Design review of the part built by this model. Coordinates are the model's own, in mm. Face numbers are marked on the shaded views. A direction names the side the tool comes from. Coordinates: 2 decimals unless noted, no trailing zeros. Loops run counter-clockwise (first coordinate to the right, second up) from the corner with the lowest first, then second, coordinate; pieces in that order, holes last. Notation, with made-up numbers: (-32.75, 68.5) -> (-19.75, 68.5) arc R23 ccw to (-19.75, 104.5) -> close; hole circle Ø6 at (82, -18). An arc over 180 degrees is marked (long way). One line per item, written item: value. Start each with the question number.
1. Insertion check: pin 1 (3 mm diameter, centred on x = -8, y = 11, fed in from -Z); pin 2 (4 mm diameter, centred on x = -7.5, y = 8.5, fed in from +Z). Each pin has a flat end and moves straight along its axis. Give the tip position at first contact, or say it passes through.
2. Draft analysis for pull direction Y (two halves, no side actions). For the marked faces 3, 4 and 5, state which applies: pulls with the +Y half, pulls with the -Y half, needs draft (parallel to the pull), parting line crosses it, or undercut.
3. For probe 1 along Y at (x, z) = (-3.75, -1.5); probe 2 along X at (y, z) = (14, -2.25); probe 3 along X at (y, z) = (18, 0.5), list the stretches that pass through material, from the lowest coordinate up.
4. Add section A-A on y = 31.5. Write out the cut boundary in (x, z).
5. Machinability: for the marked faces 1 and 2, which of the approach directions +Z, -Z, +X, -X, +Y, -Y give a long, thin tool a straight path to every point of the face, cutting with its end or side? Answer none if there is none.
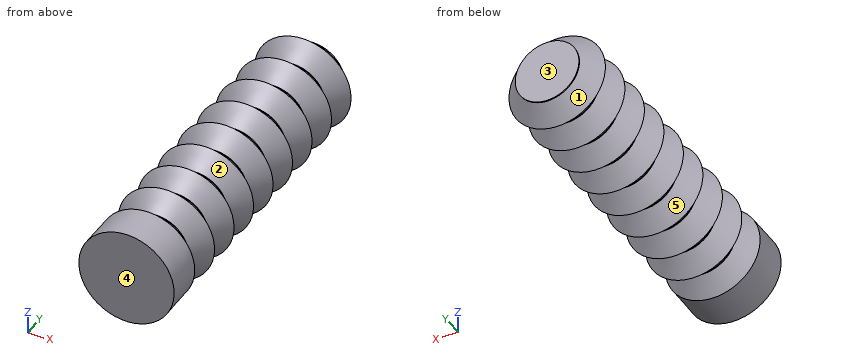
```python
from build123d import *


# Read off the part's stored shape, not the designer's step: Thicken1
with BuildPart() as part:
    # Thicken1 outline → Thicken1 (revolve)
    with BuildSketch(Plane(origin=(-5.431630681, 0, 0), x_dir=(1, 0, 0), z_dir=(0, 0, 1))):
        Polygon((0, -0.954433192), (0, -1.754433192), (4.941383818, -1.754433192), (4.918558927, 2.245501685), (3.3, 3.988409531), (3.3, 4.088409531), (5, 5.913409531), (3.3, 7.738409531), (3.3, 7.838409531), (5, 9.663409531), (3.3, 11.488409531), (3.3, 11.588409531), (5, 13.413409531), (3.3, 15.238409531), (3.3, 15.338409531), (5, 17.163409531), (3.3, 18.988409531), (3.3, 19.088409531), (5, 20.913409531), (3.3, 22.738409531), (3.3, 22.838409531), (5, 24.663409531), (3.3, 26.488409531), (3.3, 26.588409531), (5, 28.413409531), (3.3, 30.238409531), (3.3, 30.338409531), (5, 32.163409531), (3.3, 33.988409531), (3.3, 34.102954004), (0, 34.102954004), (0, 33.302954004), (2.845194483, 33.302954004), (3.906687965, 32.163409531), (2.5, 30.653288628), (2.5, 29.923530434), (3.906687965, 28.413409531), (2.5, 26.903288628), (2.5, 26.173530434), (3.906687965, 24.663409531), (2.5, 23.153288628), (2.5, 22.423530434), (3.906687965, 20.913409531), (2.5, 19.403288628), (2.5, 18.673530434), (3.906687965, 17.163409531), (2.5, 15.653288628), (2.5, 14.923530434), (3.906687965, 13.413409531), (2.5, 11.903288628), (2.5, 11.173530434), (3.906687965, 9.663409531), (2.5, 8.153288628), (2.5, 7.423530434), (3.906687965, 5.913409531), (2.5, 4.403288628), (2.5, 3.674236782), (4.120349674, 1.929400611), (4.136805741, -0.954433192), align=None)
    revolve(axis=Axis((-5.431630681, 0, 0), (0, 1, 0)))


solid = part.part
```
Worked answers:
1. pin 1: stops at z = -4.63
1. pin 2: stops at z = 4.98
2. face 3: pulls with the +Y half
2. face 4: pulls with the -Y half
2. face 5: undercut
3. probe 1: y = -1.75 to -0.95, 33.3 to 34.1
3. probe 2: x = -9.28 to -7.93, -2.94 to -1.59
3. probe 3: x = -9.62 to -8.52, -2.34 to -1.24
4. outline: circle Ø8.76 at (-5.43, 0); hole circle Ø6.58 at (-5.43, 0)
5. face 1: +Y
5. face 2: none
